```python
from build123d import *

# Parameters (mm, degrees)
ESBO_O1_W                = 45
ESBO_O1_H                = 45
BASE_DEPTH               = 1.2
ESBO_O2_W                = 5
ESBO_O2_H                = 5
PAREDES_DEPTH            = 5
ESBO_O3_W                = 45
ESBO_O3_H                = 45
TELHADO_DEPTH            = 2
CORTE_DA_BASE_DEPTH      = 2
ESBO_O5_R                = 11.25
CORTE_DO_C_RCULO_DEPTH   = 2
PONTE_1_REACH            = 48.621
ESBO_O6_W                = 5
ESBO_O6_H                = 0.8
PONTE_2_REACH            = 48.621
ESBO_O7_W                = 5
ESBO_O7_H                = 0.8
RESSALTO_EXTRUS_O6_DEPTH = 0.4
RESSALTO_EXTRUS_O7_DEPTH = 0.2
FILETE1_R                = 5
FILETE2_R                = 5
FILETE3_R                = 5
FILETE4_R                = 5


with BuildPart() as part:
    # Esboço1 → Base (new body)
    with BuildSketch(Plane(origin=(0, 0, 0), x_dir=(1, 0, 0), z_dir=(0, 1, 0))):
        Rectangle(ESBO_O1_W, ESBO_O1_H)
    extrude(amount=BASE_DEPTH)

    # Esboço2 → Paredes (add)
    with BuildSketch(Plane(origin=(0, 1.2, 0), x_dir=(1, 0, 0), z_dir=(0, 1, 0))):
        with Locations((-20, 20)):
            Rectangle(ESBO_O2_W, ESBO_O2_H)
        with Locations((20, 20)):
            Rectangle(ESBO_O2_W, ESBO_O2_H)
        with Locations((20, -20)):
            Rectangle(ESBO_O2_W, ESBO_O2_H)
        with Locations((-20, -20)):
            Rectangle(ESBO_O2_W, ESBO_O2_H)
        with Locations((0, 20)):
            Rectangle(ESBO_O2_W, ESBO_O2_H)
        with Locations((-20, 0)):
            Rectangle(ESBO_O2_W, ESBO_O2_H)
        with Locations((20, 0)):
            Rectangle(ESBO_O2_W, ESBO_O2_H)
        with Locations((0, -20)):
            Rectangle(ESBO_O2_W, ESBO_O2_H)
    extrude(amount=PAREDES_DEPTH)

    # Esboço3 → Telhado (add)
    with BuildSketch(Plane(origin=(0, 6.2, 0), x_dir=(1, 0, 0), z_dir=(0, 1, 0))):
        Rectangle(ESBO_O3_W, ESBO_O3_H)
    extrude(amount=TELHADO_DEPTH)

    # Esboço4 → Corte da Base (cut)
    with BuildSketch(Plane(origin=(0, 1.2, 0), x_dir=(1, 0, 0), z_dir=(0, 1, 0))):
        with BuildLine():
            Line((-12.5, 17.5), (12.5, 17.5))
            ThreePointArc((12.5, 17.5), (16.035533906, 16.035533906), (17.5, 12.5))
            Line((17.5, 12.5), (17.5, -12.5))
            ThreePointArc((17.5, -12.5), (16.035533906, -16.035533906), (12.5, -17.5))
            Line((12.5, -17.5), (-12.5, -17.5))
            ThreePointArc((-12.5, -17.5), (-16.035533906, -16.035533906), (-17.5, -12.5))
            Line((-17.5, -12.5), (-17.5, 12.5))
            ThreePointArc((-17.5, 12.5), (-16.035533906, 16.035533906), (-12.5, 17.5))
        make_face()
    extrude(amount=-CORTE_DA_BASE_DEPTH, mode=Mode.SUBTRACT)

    # Esboço5 → Corte do Círculo (cut)
    with BuildSketch(Plane.XZ.offset(-6.2)):
        with Locations(Location((0, 0, 0), (0, 0, 270))):
            Circle(ESBO_O5_R)
    extrude(amount=-CORTE_DO_C_RCULO_DEPTH, mode=Mode.SUBTRACT)

    # Esboço6 → Ponte 1 (add, up to next)
    with BuildSketch(Plane.XY.offset(-17.5), mode=Mode.PRIVATE) as ponte_1_sk1:
        with Locations((20, 5.8)):
            Rectangle(ESBO_O6_W, ESBO_O6_H)
    ponte_1_tool1 = extrude(ponte_1_sk1.sketch, amount=PONTE_1_REACH, mode=Mode.PRIVATE) - part.part
    # Esboço6 → Ponte 1 (add, up to next)
    with BuildSketch(Plane.XY.offset(-17.5), mode=Mode.PRIVATE) as ponte_1_sk2:
        with Locations((-20, 5.8)):
            Rectangle(ESBO_O6_W, ESBO_O6_H)
    ponte_1_tool2 = extrude(ponte_1_sk2.sketch, amount=PONTE_1_REACH, mode=Mode.PRIVATE) - part.part
    add(ponte_1_tool1.solids().sort_by_distance((20, 5.8, -17.5))[0])
    add(ponte_1_tool1.solids().sort_by_distance((20, 5.8, -17.5))[1])
    add(ponte_1_tool2.solids().sort_by_distance((-20, 5.8, -17.5))[0])
    add(ponte_1_tool2.solids().sort_by_distance((-20, 5.8, -17.5))[1])

    # Esboço7 → Ponte 2 (add, up to next)
    with BuildSketch(Plane.ZY.offset(-17.5), mode=Mode.PRIVATE) as ponte_2_sk1:
        with Locations((20, 5.8)):
            Rectangle(ESBO_O7_W, ESBO_O7_H)
    ponte_2_tool1 = extrude(ponte_2_sk1.sketch, amount=PONTE_2_REACH, mode=Mode.PRIVATE) - part.part
    # Esboço7 → Ponte 2 (add, up to next)
    with BuildSketch(Plane.ZY.offset(-17.5), mode=Mode.PRIVATE) as ponte_2_sk2:
        with Locations((-20, 5.8)):
            Rectangle(ESBO_O7_W, ESBO_O7_H)
    ponte_2_tool2 = extrude(ponte_2_sk2.sketch, amount=PONTE_2_REACH, mode=Mode.PRIVATE) - part.part
    add(ponte_2_tool1.solids().sort_by_distance((17.5, 5.8, 20))[0])
    add(ponte_2_tool1.solids().sort_by_distance((17.5, 5.8, 20))[1])
    add(ponte_2_tool2.solids().sort_by_distance((17.5, 5.8, -20))[0])
    add(ponte_2_tool2.solids().sort_by_distance((17.5, 5.8, -20))[1])

    # Esboço8 → Ressalto-extrusão6 (add)
    with BuildSketch(Plane(origin=(0, 6.2, 0), x_dir=(-1, 0, 0), z_dir=(0, -1, 0))):
        Polygon((-2, -17.5), (-17.5, -2), (-17.5, -17.5), align=None)
        Polygon((-17.5, 2), (-17.5, 17.5), (-2, 17.5), align=None)
        Polygon((2, 17.5), (17.5, 17.5), (17.5, 2), align=None)
        Polygon((17.5, -2), (17.5, -17.5), (2, -17.5), align=None)
    extrude(amount=RESSALTO_EXTRUS_O6_DEPTH)

    # Esboço10 → Ressalto-extrusão7 (add)
    with BuildSketch(Plane.XZ.offset(-6.2)):
        Polygon((-11.25, 8.25), (-11.25, -8.25), (-17.5, -2), (-17.5, 2), align=None)
        Polygon((8.25, 11.25), (2, 17.5), (-2, 17.5), (-8.25, 11.25), align=None)
        Polygon((11.25, -8.25), (17.5, -2), (17.5, 2), (11.25, 8.25), align=None)
        Polygon((-8.25, -11.25), (-2, -17.5), (2, -17.5), (8.25, -11.25), align=None)
    extrude(amount=RESSALTO_EXTRUS_O7_DEPTH)

    # Filete1
    filete1_edges = [part.edges().sort_by_distance(p)[0] for p in [
        (-22.5, 4.1, -22.5),
    ]]
    fillet(filete1_edges, radius=FILETE1_R - 0.0001)  # a hair under: the kernel refuses the full size

    # Filete2
    filete2_edges = [part.edges().sort_by_distance(p)[0] for p in [
        (-22.5, 4.1, 22.5),
    ]]
    fillet(filete2_edges, radius=FILETE2_R - 0.0001)  # a hair under: the kernel refuses the full size

    # Filete3
    filete3_edges = [part.edges().sort_by_distance(p)[0] for p in [
        (22.5, 4.1, 22.5),
    ]]
    fillet(filete3_edges, radius=FILETE3_R - 0.0001)  # a hair under: the kernel refuses the full size

    # Filete4
    filete4_edges = [part.edges().sort_by_distance(p)[0] for p in [
        (22.5, 4.1, -22.5),
    ]]
    fillet(filete4_edges, radius=FILETE4_R - 0.0001)  # a hair under: the kernel refuses the full size


solid = part.part
```
CAD build for the part. Positions are in the model's coordinates, mm. A direction names the side the tool comes from. Round coordinates to 2 decimals unless told otherwise and drop trailing zeros. Write each loop counter-clockwise with the first axis right and the second up, starting at its lowest first coordinate (ties: lowest second). Pieces come first, ordered by that corner, then holes. Notation, with made-up numbers: M 67,64 L 125,64 A23 ccw 125,102 Z; hole C 9,28.25 d8. An arc over 180 degrees is marked long. One line per question, with ' | ' between items.
1. Cut at B-B on z = 9. Write the cut outline in (x, y), and give its area (3 significant figures).
Working result:
outline: M -22.5,0 L -17.5,0 L -17.5,1.2 L -22.5,1.2 Z; M -22.5,5.4 L -17.5,5.4 L -17.5,5.8 L -10.5,5.8 L -10.5,6.2 L -6.75,6.2 L -6.75,8.2 L -22.5,8.2 Z; M 6.75,6.2 L 10.5,6.2 L 10.5,5.8 L 17.5,5.8 L 17.5,5.4 L 22.5,5.4 L 22.5,8.2 L 6.75,8.2 Z; M 17.5,0 L 22.5,0 L 22.5,1.2 L 17.5,1.2 Z | area: 88.6 mm2
2. Cut at D-D on x = -1. Write the cut outline in (y, z), and give its area (3 significant figures).
Working result:
outline: M 0,-22.5 L 8.2,-22.5 L 8.2,-11.21 L 6.2,-11.21 L 6.2,-11.25 L 6,-11.25 L 6,-17.5 L 0,-17.5 Z; M 0,17.5 L 6,17.5 L 6,11.25 L 6.2,11.25 L 6.2,11.21 L 8.2,11.21 L 8.2,22.5 L 0,22.5 Z | area: 110 mm2
3. Cut at C-C on z = 1. Write the cut outline in (x, y), and give its area (3 significant figures).
Working result:
outline: M -22.5,0 L -17.5,0 L -17.5,6 L -11.25,6 L -11.25,6.2 L -11.21,6.2 L -11.21,8.2 L -22.5,8.2 Z; M 11.21,6.2 L 11.25,6.2 L 11.25,6 L 17.5,6 L 17.5,0 L 22.5,0 L 22.5,8.2 L 11.21,8.2 Z | area: 110 mm2
4. Pin check, flat tips, straight feed: pin 1 Ø12 at (x, z) = (2, -0.5) entering from -Y; pin 2 Ø2 at (y, z) = (3.5, -21) entering from -X; pin 3 Ø1.3 at (x, y) = (-20, 4) entering from -Z; pin 4 Ø3 at (x, z) = (-15.5, -2.5) entering from -Y. Stop position of each tip, or through.
Working result:
pin 1: through | pin 2: x = -21.83 | pin 3: z = -22.15 | pin 4: y = 5.8
5. Cut at A-A on x = -16.5. Write the cut outline in (y, z), and give its area (3 significant figures).
Working result:
outline: M 0,-22.5 L 1.2,-22.5 L 1.2,-15.5 L 0,-15.5 Z; M 0,15.5 L 1.2,15.5 L 1.2,22.5 L 0,22.5 Z; M 5.4,-22.5 L 8.2,-22.5 L 8.2,22.5 L 5.4,22.5 L 5.4,17.5 L 5.8,17.5 L 5.8,3 L 6,3 L 6,-3 L 5.8,-3 L 5.8,-17.5 L 5.4,-17.5 Z | area: 128 mm2
6. Mould opens along X. For faces 4 (the flat face through (20, 3, 2.5)), 5 (the flat face through (13, 5.8, 13)) say: pulls with the +X half, pulls with the -X half, needs draft (parallel to the pull), parting line crosses it, or undercut.
Working result:
face 4: needs draft | face 5: undercut
7. Which spindle directions (+Z, -Z, +X, -X, +Y, -Y) get a long thin tool onto all of the face, cutting with end or side? Do faces 1 (the flat face through (-2.5, 3, -20)), 2 (the flat face through (20, 5.4, 10)), 3 (the cylindrical face through (16, 0.61, -16.07)). Say none if no direction does.
Working result:
face 1: +Z, -Z | face 2: +X, -X | face 3: -Y
8. Probe L1, parallel to X at y = 6.9, z = 0; L2, parallel to X at y = 0.5, z = 10. List the from-to ranges inside material, lowest first. Write a range as from..to.
Working result:
L1: -22.5..-11.25, 11.25..22.5 | L2: -22.5..-17.5, 17.5..22.5
